Check sheet for the modelled part. Datum: model origin and axes. Units: mm. Give positions to 0.01 mm unless a question says otherwise; leave off trailing zeros. Order: outer loops, then holes, each group sorted by start corner. A loop starts at its lowest first (then second) coordinate and runs counter-clockwise, first axis right, second up. Notation, with made-up numbers: (-14.75, 12) - (31.25, 12) arc R27 cw to (31.25, 29) - close; hole circle Ø8 at (62, 63.5). An arc over 180 degrees is marked (long way). Answer in a Markdown table with one row per item.
from build123d import *

# Parameters (mm, degrees)
BOSS_EXTRUDE1_DEPTH = 9.525
FILLET1_R           = 0.635


with BuildPart() as part:
    # Sketch1 → Boss-Extrude1 (new body)
    with BuildSketch(Plane(origin=(0, 0, 0), x_dir=(0, 0, -1), z_dir=(1, 0, 0))):
        Polygon((-6.35, 17.4625), (-3.175, 20.6375), (6.35, 20.6375), (6.35, 17.4625), (6.35, -17.4625), (-6.35, -17.4625), align=None)
    extrude(amount=BOSS_EXTRUDE1_DEPTH)

    # Fillet1
    fillet1_edges = [part.edges().sort_by_distance(p)[0] for p in [
        (4.7625, -17.4625, -6.35),
        (4.7625, -17.4625, 6.35),
        (4.7625, 17.4625, 6.35),
        (4.7625, 20.6375, 3.175),
        (4.7625, 20.6375, -6.35),
    ]]
    fillet(fillet1_edges, radius=FILLET1_R)


solid = part.part
(1) Mould release check, pull along Z, two halves, no side actions. Record for faces 1 (the flat face through (0, 2, 0)), 2 (the flat face through (5, 0, 6.35)), 3 (the flat face through (5, 1, -6.35)): pulls with the +Z half, pulls with the -Z half, needs draft (parallel to the pull), parting line crosses it, or undercut.
Geometry says:
| item | result |
|---|---|
| face 1 | needs draft |
| face 2 | pulls with the +Z half |
| face 3 | pulls with the -Z half |
(2) Cross-section at A-A, the plane z = 4.5. Record the cut outline in (x, y) (1 decimal).
Geometry says:
| item | result |
|---|---|
| outline | (0, -17.5) - (9.5, -17.5) - (9.5, 19.3) - (0, 19.3) - close |
(3) Thickness scan on L1, parallel to Y at x = 4.5, z = 4.5; L2, parallel to Z at x = 4.25, y = 19; L3, parallel to Y at x = 7.25, z = 5.25. Record the ranges inside material, lowest first.
Geometry says:
| item | result |
|---|---|
| L1 | -17.46 to 19.31 |
| L2 | -6.35 to 4.81 |
| L3 | -17.46 to 18.56 |
